For this review, take the finished solid that the model builds, in its own axes (mm). Face numbers are marked on the shaded views. A direction names the side the tool comes from. Give positions to 0.01 mm unless a question says otherwise; leave off trailing zeros. Write each loop counter-clockwise with the first axis right and the second up, starting at its lowest first coordinate (ties: lowest second). Pieces come first, ordered by that corner, then holes.
Q1. We need section B-B (y = 0). Write out the cut boundary in (x, z), then the cut area to 3 significant figures.
Q2. We need section D-D (x = 17). Write out the cut boundary in (y, z).
Q3. For line 1 (Y direction, x = 0, z = 26.5); line 2 (Z direction, x = -14, y = -22); line 3 (Y direction, x = 13, z = 14.5), list the stretches that pass through material, from the lowest coordinate up.
Q4. We need section A-A (z = 12). Write out the cut boundary in (x, y).
Q5. Machinability: for the marked faces 1 and 2, which of the approach directions +Z, -Z, +X, -X, +Y, -Y give a long, thin tool a straight path to every point of the face, cutting with its end or side? Answer none if there is none.
Q6. Mouldability with a two-part tool opening along X and no side actions: class the marked faces 3 and 4 as released by +X, released by -X, zero draft, split by the parting line, or undercut.
Q7. We need section C-C (x = -5). Write out the cut boundary in (y, z).
Q8. Insertion check: P1, Ø4, axis at y = -24.5, z = 31.5, coming from the +X side; P2, Ø3, axis at x = -4.5, y = 8.5, coming from the +Z side; P3, Ø2.5, axis at y = 24.5, z = 30, coming from the -X side. Each pin has a flat end and moves straight along its axis. Give the tip position at first contact, or say it passes through.
```python
from build123d import *

# Parameters (mm, degrees)
SKETCH1_R           = 35.55
SKETCH1_R_2         = 32.55
BOSS_EXTRUDE1_DEPTH = 47
BOSS_EXTRUDE2_START = 2
SKETCH2_R           = 35.55
BOSS_EXTRUDE2_DEPTH = 2
SKETCH4_R           = 32.55
SKETCH4_R_2         = 30
BOSS_EXTRUDE3_DEPTH = 38
CUT_EXTRUDE1_START  = -42
CUT_EXTRUDE1_DEPTH  = 42


with BuildPart() as part:
    # Sketch1 → Boss-Extrude1 (new body)
    with BuildSketch(Plane.XY):
        Circle(SKETCH1_R)
        Circle(SKETCH1_R_2, mode=Mode.SUBTRACT)
    extrude(amount=BOSS_EXTRUDE1_DEPTH)

    # Sketch2 → Boss-Extrude2 (add)
    with BuildSketch(Plane(origin=(0, 0, 0), x_dir=(-1, 0, 0), z_dir=(0, 0, -1)).offset(BOSS_EXTRUDE2_START)):
        Circle(SKETCH2_R)
    extrude(amount=-BOSS_EXTRUDE2_DEPTH)

    # Sketch4 → Boss-Extrude3 (add)
    with BuildSketch(Plane.XY):
        Circle(SKETCH4_R)
        Circle(SKETCH4_R_2, mode=Mode.SUBTRACT)
    extrude(amount=BOSS_EXTRUDE3_DEPTH)

    # Sketch5 → Cut-Extrude1 (cut)
    with BuildSketch(Plane.XY.offset(47).offset(CUT_EXTRUDE1_START)):
        with BuildLine():
            Line((-35.55, 35.55), (-35.55, -3.6e-08))
            ThreePointArc((-35.55, -3.6e-08), (-31.978075564, 15.530781797), (-21.980088117, 27.940619649))
            Line((-21.980088117, 27.940619649), (-21.980088117, 35.55))
            Line((-21.980088117, 35.55), (-35.55, 35.55))
        make_face()
        with BuildLine():
            ThreePointArc((-21.980088117, 27.940619649), (-31.978075564, 15.530781797), (-35.55, -3.6e-08))
            ThreePointArc((-35.55, -3.6e-08), (-31.978075549, -15.530781829), (-21.980088117, -27.940619649))
            Line((-21.980088117, -27.940619649), (-21.980088117, -24.007878423))
            ThreePointArc((-21.980088117, -24.007878423), (-32.55, 0), (-21.980088117, 24.007878423))
            Line((-21.980088117, 24.007878423), (-21.980088117, 27.940619649))
        make_face()
        with BuildLine():
            ThreePointArc((-21.980088117, 24.007878423), (-32.55, 0), (-21.980088117, -24.007878423))
            Line((-21.980088117, -24.007878423), (-21.980088117, 24.007878423))
        make_face()
        with BuildLine():
            Line((-35.55, -3.6e-08), (-35.55, -35.55))
            Line((-35.55, -35.55), (-21.980088117, -35.55))
            Line((-21.980088117, -35.55), (-21.980088117, -27.940619649))
            ThreePointArc((-21.980088117, -27.940619649), (-31.978075549, -15.530781829), (-35.55, -3.6e-08))
        make_face()
        with BuildLine():
            Line((21.980088117, -27.940619649), (21.980088117, -35.55))
            Line((21.980088117, -35.55), (35.55, -35.55))
            Line((35.55, -35.55), (35.55, 0))
            ThreePointArc((35.55, 0), (31.978075556, -15.530781813), (21.980088117, -27.940619649))
        make_face()
        with BuildLine():
            Line((21.980088117, -24.007878423), (21.980088117, -27.940619649))
            ThreePointArc((21.980088117, -27.940619649), (31.978075556, -15.530781813), (35.55, 0))
            ThreePointArc((35.55, 0), (31.978075556, 15.530781813), (21.980088117, 27.940619649))
            Line((21.980088117, 27.940619649), (21.980088117, 24.007878423))
            ThreePointArc((21.980088117, 24.007878423), (29.790555284, 13.115842172), (32.55, 0))
            ThreePointArc((32.55, 0), (29.790555284, -13.115842172), (21.980088117, -24.007878423))
        make_face()
        with BuildLine():
            Line((21.980088117, 24.007878423), (21.980088117, -24.007878423))
            ThreePointArc((21.980088117, -24.007878423), (29.790555284, -13.115842172), (32.55, 0))
            ThreePointArc((32.55, 0), (29.790555284, 13.115842172), (21.980088117, 24.007878423))
        make_face()
        with BuildLine():
            ThreePointArc((21.980088117, 27.940619649), (31.978075556, 15.530781813), (35.55, 0))
            Line((35.55, 0), (35.55, 35.55))
            Line((35.55, 35.55), (21.980088117, 35.55))
            Line((21.980088117, 35.55), (21.980088117, 27.940619649))
        make_face()
    extrude(amount=CUT_EXTRUDE1_DEPTH, mode=Mode.SUBTRACT)


solid = part.part
```
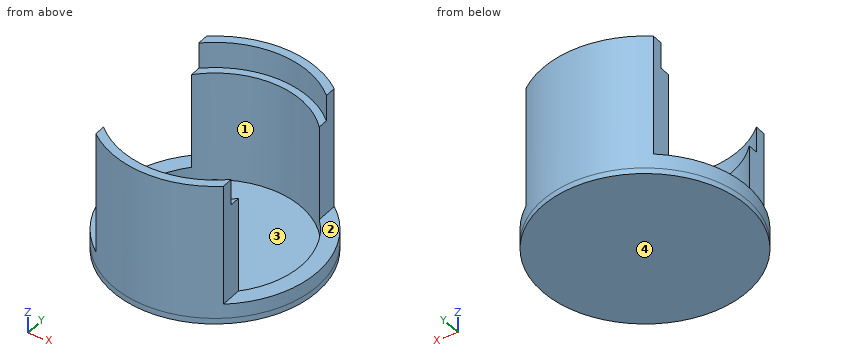
Computed:
1. outline: (-35.55, -2) - (35.55, -2) - (35.55, 5) - (30, 5) - (30, 0) - (-30, 0) - (-30, 5) - (-35.55, 5) - close
1. area: 198 mm2
2. outline: (-31.22, -2) - (31.22, -2) - (31.22, 47) - (27.76, 47) - (27.76, 38) - (24.72, 38) - (24.72, 0) - (-24.72, 0) - (-24.72, 38) - (-27.76, 38) - (-27.76, 47) - (-31.22, 47) - close
3. line 1: y = -35.55 to -30, 30 to 35.55
3. line 2: z = -2 to 0
3. line 3: y = -33.09 to -27.04, 27.04 to 33.09
4. outline: (-21.98, -27.94) arc R35.55 ccw to (21.98, -27.94) - (21.98, -20.42) arc R30 cw to (-21.98, -20.42) - close; (-21.98, 20.42) arc R30 cw to (21.98, 20.42) - (21.98, 27.94) arc R35.55 ccw to (-21.98, 27.94) - close
5. face 1: +Z
5. face 2: +Z, +X, +Y, -Y
6. face 3: undercut
6. face 4: zero draft
7. outline: (-35.2, -2) - (35.2, -2) - (35.2, 47) - (32.16, 47) - (32.16, 38) - (29.58, 38) - (29.58, 0) - (-29.58, 0) - (-29.58, 38) - (-32.16, 38) - (-32.16, 47) - (-35.2, 47) - close
8. P1: stops at x = 21.98
8. P2: stops at z = 0
8. P3: stops at x = -21.98
